Autodesk Inventor part; units mm, degrees
ref_plane "Płaszczyzna konstrukcyjna1" through (-9.4999, -9.4999, 27.64) normal (0, 0, 1) x (0.8774, -0.4797, 0)
ref_plane "Płaszczyzna konstrukcyjna2" through (-6.6123, -6.6123, 155) normal (0, 0, -1) x (-0.1077, 0.9942, 0)
ref_plane "YZ Plane" through (0, 0, 0) normal (1, 0, 0) x (0, 1, 0)
sketch "Sketch1" plane through (0, 0, 0) normal (0, 0, 1) x (1, 0, 0)
  circle A0 centre (0, 0) radius 7.5
  circle A1 centre (0, 0) radius 5.5
  circle A2 centre (0, 0) radius 5
extrude "Extrusion1" add sketch "Sketch1" against normal blind 50 contours A2
sketch "Sketch2" plane through (0, 0, 0) normal (0, 0, 1) x (1, 0, 0)
  point P0 (0, 0)
sketch "Sketch3" plane through (0, 0, 0) normal (0, 0, 1) x (1, 0, 0)
  circle A0 centre (0, 0) radius 5
extrude "Extrusion2" add sketch "Sketch3" along normal blind 150
sketch "Sketch4" plane through (0, 0, 150) normal (0, 0, 1) x (1, 0, 0)
  circle A0 centre (0, 0) radius 5
  circle A1 centre (0, 0) radius 4
  dimension "d4" = 8
extrude "Extrusion3" cut sketch "Sketch4" against normal blind 30
sketch "Sketch5" plane through (0, 0, -50) normal (0, 0, -1) x (-1, 0, 0)
  circle A0 centre (0, 0) radius 5
extrude "Extrusion4" add sketch "Sketch5" along normal blind 20
sketch "Szkic6" plane through (0, 0, -70) normal (0, 0, -1) x (-1, 0, 0)
  circle A0 centre (0, 0) radius 4
  circle A1 centre (0, 0) radius 5
extrude "Wyciągnięcie proste5" add sketch "Szkic6" along normal blind 6 contours A0 | A1
sketch "Szkic7" plane through (0, 0, 150) normal (0, 0, 1) x (1, 0, 0)
  circle A0 centre (0, 0) radius 5
  circle A1 centre (0, 0) radius 5
ref_plane "Płaszczyzna konstrukcyjna1" through (-9.4999, -9.4999, 27.64) normal (0, 0, 1) x (0.8774, -0.4797, 0)
extrude "Wyciągnięcie proste6" cut sketch "Szkic7" against normal up to surface (122.36 mm away)
sketch "Szkic8" plane through (0, 0, 27.64) normal (0, 0, 1) x (1, 0, 0)
  circle A0 centre (0, 0) radius 5
  circle A1 centre (0, 0) radius 4.4644
  point P0 (0, 0)
extrude "Wyciągnięcie proste7" add sketch "Szkic8" along normal blind 2 contours A1
sketch "Szkic9" plane through (0, 0, 29.64) normal (0, 0, 1) x (1, 0, 0)
  circle A0 centre (0, 0) radius 4.4644
  circle A1 centre (0, 0) radius 5
  point P0 (0, 0)
ref_plane "Płaszczyzna konstrukcyjna2" through (-6.6123, -6.6123, 155) normal (0, 0, -1) x (-0.1077, 0.9942, 0)
extrude "Wyciągnięcie proste8" add sketch "Szkic9" along normal up to surface (125.36 mm away) contours A0 | A1
sketch "Szkic10" plane through (0, 0, -76) normal (0, 0, -1) x (-1, 0, 0)
  circle A0 centre (0, 0) radius 5
  point P0 (0, 0)
extrude "Wyciągnięcie proste9" add sketch "Szkic10" along normal blind 15
sketch "Szkic11" plane through (0, 0, 27.64) normal (0, 0, 1) x (1, 0, 0)
  circle A0 centre (0, 0) radius 5
  circle A1 centre (0, 0) radius 4.4644
  circle A2 centre (0, 0) radius 6
  point P0 (0, 0)
  dimension "d19" = 12
extrude "Wyciągnięcie proste10" add sketch "Szkic11" along normal blind 97.36 contours A0 | A1 | A2
sketch "Szkic12" plane through (0, 0, -91) normal (0, 0, -1) x (-1, 0, 0)
  circle A0 centre (0, 0) radius 5
  point P0 (0, 0)
extrude "Wyciągnięcie proste11" cut sketch "Szkic12" against normal blind 0.6
sketch "Szkic13" plane through (0, 0, -90.4) normal (0, 0, -1) x (-1, 0, 0)
  circle A0 centre (0, 0) radius 5
extrude "Wyciągnięcie proste12" cut sketch "Szkic13" against normal blind 0.04
sketch "Szkic14" plane through (0, 0, 125) normal (0, 0, 1) x (1, 0, 0)
  circle A0 centre (0, 0) radius 6
  circle A1 centre (0, 0) radius 5
  point P0 (0, 0)
extrude "Wyciągnięcie proste13" cut sketch "Szkic14" against normal blind 0.36
sketch "Szkic15" plane through (0, 0, 155) normal (0, 0, 1) x (1, 0, 0)
  circle A0 centre (0, 0) radius 5
  point P0 (0, 0)
extrude "Wyciągnięcie proste14" cut sketch "Szkic15" against normal blind 0.36
properties part number "os_napedowa"
Geometry check sheet. Reference: the model listing, model coordinates, mm. A direction names the side the tool comes from. Round coordinates to 2 decimals unless told otherwise and drop trailing zeros. Loops run counter-clockwise (first coordinate to the right, second up) from the corner with the lowest first, then second, coordinate; pieces in that order, holes last. Notation, with made-up numbers: (24.25, 72.5) - (59.25, 72.5) arc R28 ccw to (59.25, 96.5) - close; hole circle Ø10 at (-32, 62.25). An arc over 180 degrees is marked (long way). Use a Markdown table: item, result.
Q1. Cross-section at C-C on z = 133. Record the cut outline in (x, y).
Solutions:
| item | result |
|---|---|
| outline | circle Ø10 at (0, 0) |
Q2. Cross-section at D-D on z = 90. Record the cut outline in (x, y).
Solutions:
| item | result |
|---|---|
| outline | circle Ø12 at (0, 0) |
Q3. Go/stop test with flat-tipped pins: P1, Ø4, axis at x = 0.5, z = 109, coming from the -Y side; P2, Ø3, axis at y = 4.5, z = 92, coming from the -X side; P3, Ø4, axis at x = 1.5, z = 3.5, coming from the -Y side; P4, Ø1.5, axis at x = -2, z = -46.5, coming from the -Y side. Record where each tip stops, or that it passes through.
Solutions:
| item | result |
|---|---|
| P1 | stops at y = -6 |
| P2 | stops at x = -5.2 |
| P3 | stops at y = -5 |
| P4 | stops at y = -4.84 |
Q4. Access from +Z, -Z, +X, -X, +Y, -Y to the whole of each face (thin tool, end or side, straight path). Record for faces 1 (the flat face through (-4, 4, 27.64)), 2 (the flat face through (-4, 4, 124.64)), 3 (the flat face through (0, 0, -90.36)).
Solutions:
| item | result |
|---|---|
| face 1 | -Z |
| face 2 | +Z |
| face 3 | -Z, +X, -X, +Y, -Y |
Q5. Cross-section at A-A on x = 0. Record the cut outline in (y, z).
Solutions:
| item | result |
|---|---|
| outline | (-6, 27.64) - (-5, 27.64) - (-5, -90.36) - (5, -90.36) - (5, 27.64) - (6, 27.64) - (6, 124.64) - (5, 124.64) - (5, 154.64) - (-5, 154.64) - (-5, 124.64) - (-6, 124.64) - close |
Q6. Material ranges on line 1 (Y direction, x = -0.25, z = 48.5); line 2 (Y direction, x = -0.25, z = 17.5); line 3 (Z direction, x = 4.75, y = -2), recorded low to high.
Solutions:
| item | result |
|---|---|
| line 1 | y = -5.99 to 5.99 |
| line 2 | y = -4.99 to 4.99 |
| line 3 | z = 27.64 to 124.64 |
